Source: CAD feature listing. Evaluate the final solid. Frame: model axes, mm. Face numbers are marked on the shaded views. A direction names the side the tool comes from. Give positions to 0.01 mm unless a question says otherwise; leave off trailing zeros. Order: outer loops, then holes, each group sorted by start corner. A loop starts at its lowest first (then second) coordinate and runs counter-clockwise, first axis right, second up.
1) Section A-A, the plane y = 0. Return loops of the section in (x, z), plus the area to 3 significant figures.
2) Section D-D, the plane x = 9.75. Return loops of the section in (y, z).
3) Section C-C, the plane z = 5.5. Return loops of the section in (x, y), plus the area to 3 significant figures.
4) Section B-B, the plane x = -5.5. Return loops of the section in (y, z).
5) Access query for the marked faces 1 and 2. Directions: +Z, -Z, +X, -X, +Y, -Y. A direction counts if a zero-diameter tool reaches every point of the face in a straight line with its end or side. Return the directions, or none.
6) Draft query along X for the marked faces 3, 4 and 5. Return one class per face: released by +X, released by -X, zero draft, split by the parting line, or undercut.
7) First-contact query: P1, Ø4, axis at y = -0.5, z = 4, coming from the -X side; P2, Ø3, axis at y = -3.5, z = 3, coming from the -X side; P3, Ø5, axis at y = -3, z = 3.5, coming from the +X side; P4, Ø1.5, axis at y = -5.5, z = 8.5, coming from the -X side. Flat tips, straight axial feed; report the tip coordinate or a pass-through.
8) Material intervals for line 1 (X direction, y = -6.25, z = 5); line 2 (Y direction, x = -1.75, z = 2.75); line 3 (Y direction, x = 4.75, z = 7.5), sorted ascending.
```python
from build123d import *

# Parameters (mm, degrees)
F0_R     = 13.1191
F1_DEPTH = 12.7
F3_DEPTH = 36.322


# Not quite as in the source:
# - a length typed as a fraction of an inch, garbled in the dataset ("3 / 203.2 mm" for 3/8 in), is restored


with BuildPart() as f1:
    # F0 (on Top) → F1 (new body)
    with BuildSketch(Plane.XY):
        Circle(F0_R)
    extrude(amount=F1_DEPTH)

    # F2 (on Top) → F3 (cut)
    with BuildSketch(Plane.XY):
        Polygon((6.604, -3.8128211777), (6.604, 3.8128211777), (0, 7.6256423555), (-6.604, 3.8128211777), (-6.604, -3.8128211777), (0, -7.6256423555), align=None)
    extrude(amount=F3_DEPTH, mode=Mode.SUBTRACT)


solid = f1.part
```
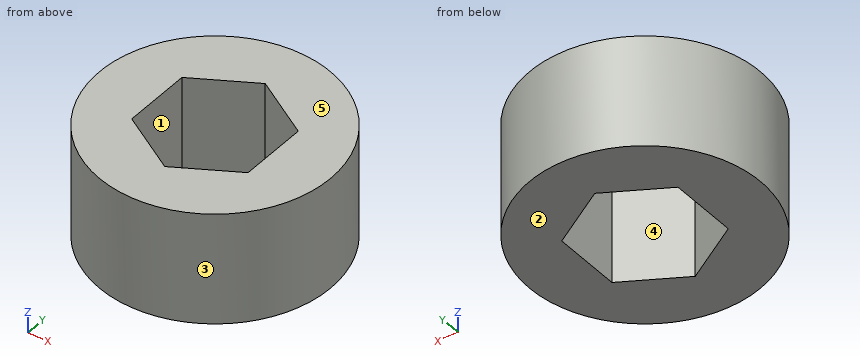
From the geometry:
1. outline: (-13.12, 0) - (-6.6, 0) - (-6.6, 12.7) - (-13.12, 12.7) - close; (6.6, 0) - (13.12, 0) - (13.12, 12.7) - (6.6, 12.7) - close
1. area: 165 mm2
2. outline: (-8.78, 0) - (8.78, 0) - (8.78, 12.7) - (-8.78, 12.7) - close
3. outline: circle Ø26.24 at (0, 0); hole (-6.6, -3.81) - (0, -7.63) - (6.6, -3.81) - (6.6, 3.81) - (0, 7.63) - (-6.6, 3.81) - close
3. area: 390 mm2
4. outline: (-11.91, 0) - (-4.45, 0) - (-4.45, 12.7) - (-11.91, 12.7) - close; (4.45, 0) - (11.91, 0) - (11.91, 12.7) - (4.45, 12.7) - close
5. face 1: +Z, -Z
5. face 2: -Z, +X, -X, +Y, -Y
6. face 3: split by the parting line
6. face 4: undercut
6. face 5: zero draft
7. P1: stops at x = -13.12
7. P2: stops at x = -12.97
7. P3: stops at x = 13.11
7. P4: stops at x = -12.23
8. line 1: x = -11.53 to -2.38, 2.38 to 11.53
8. line 2: y = -13 to -6.62, 6.62 to 13
8. line 3: y = -12.23 to -4.88, 4.88 to 12.23
